```python
from build123d import *

# Parameters (mm, degrees)
BOSS_EXTRUDE1_DEPTH = 15.2
SKETCH2_R           = 6
BOSS_EXTRUDE2_DEPTH = 12.5
SKETCH3_W           = 16
SKETCH3_H           = 28
BOSS_EXTRUDE3_DEPTH = 19
FILLET1_R           = 3
FILLET2_R           = 2


with BuildPart() as part:
    # Sketch1 → Boss-Extrude1 (new body)
    with BuildSketch(Plane(origin=(0, 0, 0), x_dir=(0, 0, -1), z_dir=(1, 0, 0))):
        Polygon((0, 0), (-40, 0), (0, 35), align=None)
    extrude(amount=BOSS_EXTRUDE1_DEPTH)

    # Sketch2 → Boss-Extrude2 (add)
    with BuildSketch(Plane.XZ):
        with Locations((7.6, 13)):
            Circle(SKETCH2_R)
    extrude(amount=BOSS_EXTRUDE2_DEPTH)

    # Sketch3 → Boss-Extrude3 (add)
    with BuildSketch(Plane.XZ.offset(12.5)):
        with Locations((7.6, 14)):
            Rectangle(SKETCH3_W, SKETCH3_H)
    extrude(amount=BOSS_EXTRUDE3_DEPTH)

    # Fillet1
    fillet1_edges = [part.edges().sort_by_distance(p)[0] for p in [
        (7.6, 35, 0),
    ]]
    fillet(fillet1_edges, radius=FILLET1_R)

    # Fillet2
    fillet2_edges = [part.edges().sort_by_distance(p)[0] for p in [
        (0, 15.323212702, 22.487756912),
        (15.2, 15.323212702, 22.487756912),
        (0, 31.120594062, 1.760351153),
        (15.2, 31.120594062, 1.760351153),
        (15.2, 14.19434766, 0),
        (0, 14.19434766, 0),
        (7.6, 0, 0),
        (7.6, 0, 40),
    ]]
    fillet(fillet2_edges, radius=FILLET2_R)


solid = part.part
```
Design review of the part built by this model. Coordinates are the model's own, in mm. A direction names the side the tool comes from. Coordinates: 2 decimals unless noted, no trailing zeros. Order: outer loops, then holes, each group sorted by start corner. A loop starts at its lowest first (then second) coordinate and runs counter-clockwise, first axis right, second up. Notation, with made-up numbers: (3, -18) - (50, -18) arc R31 cw to (50, 15) - close; hole circle Ø7 at (-36, 38). An arc over 180 degrees is marked (long way). Answer in a Markdown table with one row per item.
(1) Consider section B-B on y = -1.5. State the section outline as (x, z) points.
Checked values:
| item | result |
|---|---|
| outline | circle Ø12 at (7.6, 13) |
(2) Consider section A-A on x = 7.6. State the section outline as (y, z) points, plus the area to 3 significant figures.
Checked values:
| item | result |
|---|---|
| outline | (-31.5, 0) - (-12.5, 0) - (-12.5, 7) - (0, 7) - (0, 2) arc R2 ccw to (2, 0) - (28.39, 0) arc R3 ccw to (30.65, 4.98) - (3.51, 35.99) arc R2 ccw to (0, 34.68) - (0, 19) - (-12.5, 19) - (-12.5, 28) - (-31.5, 28) - close |
| area | 1,370 mm^2 |
(3) For faces 1 (the flat face through (7, 0, 22)), 2 (the flat face through (15.2, 12, 15)), 3 (the flat face through (7, -22, 28)), list the 3-axis set-ups (+Z, -Z, +X, -X, +Y, -Y) from which the entire face can be reached by the end or side of a thin tool; tool diameter is ignored.
Checked values:
| item | result |
|---|---|
| face 1 | none |
| face 2 | +Z, -Z, +X, +Y |
| face 3 | +Z, +X, -X, -Y |
(4) Wall thickness on line 1 along Z through (x, y) = (14.25, -14.5); line 2 along Y through (x, z) = (8.25, 20); line 3 along Y through (x, z) = (2.5, 25) (3 decimals): over which ranges is each line inside the solid? List them lowest first. Write a range as from..to.
Checked values:
| item | result |
|---|---|
| line 1 | 0..28 |
| line 2 | -31.5..-12.5, 0..17.5 |
| line 3 | -31.5..-12.5, 0..13.125 |
(5) Consider section C-C on y = -20.5. State the section outline as (x, z) points.
Checked values:
| item | result |
|---|---|
| outline | (-0.4, 0) - (15.6, 0) - (15.6, 28) - (-0.4, 28) - close |
(6) Clearance check with flat-ended pins moving along their axes: pin 1 (5 mm diameter, centred on y = 10.5, z = 25.5, fed in from +X); pin 2 (8 mm diameter, centred on x = 7.5, z = 19.5, fed in from +Y); pin 3 (3 mm diameter, centred on y = 24, z = 13, fed in from -X); pin 4 (5 mm diameter, centred on x = 3.5, y = -16.5, fed in from -Z). State where each tip first meets the part, or that it passes through.
Checked values:
| item | result |
|---|---|
| pin 1 | x = 15.2 |
| pin 2 | y = 21.44 |
| pin 3 | x = 0.16 |
| pin 4 | z = 0 |
